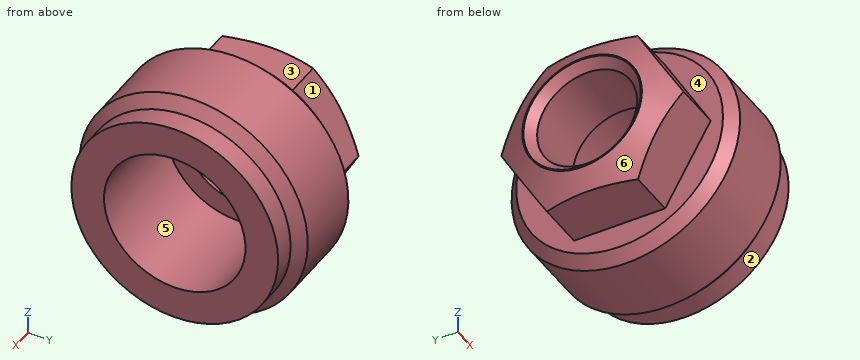
from build123d import *

# Parameters (mm, degrees)
CUT_EXTRUDE_START   = -12
SKETCH_2_R          = 17.5
CUT_EXTRUDE_1_DEPTH = 12
CHAMFER_1_SIZE      = 2
CHAMFER_2_SIZE      = 1.6


with BuildPart() as part:
    # Эскиз1 → Повернуть1 (revolve)
    with BuildSketch(Plane.XY, mode=Mode.PRIVATE) as revolve_1_sk:
        Polygon((0, -9.188), (0, -11), (3.75277675, -17.5), (12, -17.5), (12, -21), (27, -21), (29, -19), (33, -19), (33, -13), (13, -13), (13, -9.188), align=None)
    revolve(revolve_1_sk.sketch.rotate(Axis((0, 0, 0), (1, 0, 0)), 270), axis=Axis((0, 0, 0), (1, 0, 0)))

    # Эскиз2 → Вырез-Вытянуть1 (cut)
    with BuildSketch(Plane.ZY.offset(CUT_EXTRUDE_START)):
        Circle(SKETCH_2_R)
        Polygon((0, 16.743157806), (-14.5, 8.371578903), (-14.5, -8.371578903), (0, -16.743157806), (14.5, -8.371578903), (14.5, 8.371578903), align=None, mode=Mode.SUBTRACT)
    extrude(amount=CUT_EXTRUDE_1_DEPTH, mode=Mode.SUBTRACT)

    # Фаска1
    chamfer_1_edges = [part.edges().sort_by_distance(p)[0] for p in [
        (12, 0, -21),
    ]]
    chamfer(chamfer_1_edges, length=CHAMFER_1_SIZE)

    # Фаска2
    chamfer_2_edges = [part.edges().sort_by_distance(p)[0] for p in [
        (0, 0, -9.188),
    ]]
    chamfer(chamfer_2_edges, length=CHAMFER_2_SIZE)


solid = part.part
Here's how the part is built. I have some questions about the finished solid (model axes, mm). Face numbers are marked on the shaded views. A direction names the side the tool comes from. Coordinates: 2 decimals unless noted, no trailing zeros. Order: outer loops, then holes, each group sorted by start corner. A loop starts at its lowest first (then second) coordinate and runs counter-clockwise, first axis right, second up. Notation, with made-up numbers: (10.25, 29) - (52.25, 29) arc R17 cw to (52.25, 57) - close; hole circle Ø7 at (40, -18.5). An arc over 180 degrees is marked (long way). Use CSV: the item, a comma, the result in double quotes. Start each with the question number.
1. I'm going to push flat-ended pins straight in: pin 1 (24 mm diameter, centred on y = 0, z = 0, fed in from +X); pin 2 (8 mm diameter, centred on x = 5, y = 0, fed in from +Z); pin 3 (1 mm diameter, centred on y = 17, z = 11.5, fed in from -X). Where does each tip first touch, or does it pass through?
2. Suppose I cut it at A-A on y = 0. List the corners of the cut face in (x, z) for me, then the cut area to 3 significant figures.
3. If we mould it in two halves opening along Z, with no side actions, what happens to the marked faces 4, 5 and 6? For each: +Z half, -Z half, draft (parallel to the pull), parting line (faces both ways), or undercut.
4. Suppose I cut it at C-C on x = 21. List the corners of the cut face in (y, z) for me.
5. Please list where these lines run through material, in increasing order: line 1 (Y direction, x = 20, z = 0); line 2 (X direction, y = -3, z = 17); line 3 (Y direction, x = 23, z = -4.5). Write a range as from..to.
6. For the marked faces 1, 2 and 3, which set-ups out of +Z, -Z, +X, -X, +Y, -Y let a thin tool reach every point of the face, with its end or its side?
7. Suppose I cut it at B-B on x = 9. List the corners of the cut face in (y, z) for me, then the cut area to 3 significant figures.
Output:
1,pin 1,"stops at x = 13"
1,pin 2,"stops at z = 14.5"
1,pin 3,"stops at x = 13.02"
2,outline,"(0, -11) - (2.02, -14.5) - (12, -14.5) - (12, -19) - (14, -21) - (27, -21) - (29, -19) - (33, -19) - (33, -13) - (13, -13) - (13, -9.19) - (1.6, -9.19) - (0, -10.79) - close; (0, 10.79) - (1.6, 9.19) - (13, 9.19) - (13, 13) - (33, 13) - (33, 19) - (29, 19) - (27, 21) - (14, 21) - (12, 19) - (12, 14.5) - (2.02, 14.5) - (0, 11) - close"
2,area,"437 mm2"
3,face 4,"draft"
3,face 5,"undercut"
3,face 6,"parting line"
4,outline,"circle Ø42 at (0, 0); hole circle Ø26 at (0, 0)"
5,line 1,"y = -21..-13, 13..21"
5,line 2,"x = 12..33"
5,line 3,"y = -20.51..-12.2, 12.2..20.51"
6,face 1,"+Z, -X, +Y"
6,face 2,"+X"
6,face 3,"+Z, -X, +Y, -Y"
7,outline,"(-16.74, 0) - (-8.37, -14.5) - (8.37, -14.5) - (16.74, 0) - (8.37, 14.5) - (-8.37, 14.5) - close; hole circle Ø18.38 at (0, 0)"
7,area,"463 mm2"
